from build123d import *

# Parameters (mm, degrees)
BOSS_EXTRUDE1_DEPTH = 3
FILLET4_R           = 0.7
FILLET5_R           = 4.8


with BuildPart() as part:
    # Sketch1 → Boss-Extrude1 (new body)
    with BuildSketch(Plane(origin=(0, 0, 0), x_dir=(1, 0, 0), z_dir=(0, 1, 0))):
        Polygon((-25, -25), (25, -25), (25, 20.2), (20.2, 20.2), (20.2, 3.75), (16.600191324, 3.712885357), (16.528023963, 10.712513338), (13.028209972, 10.676429657), (8.674837116, 6.131306471), (8.798552593, -5.868055782), (13.244712056, -10.322454286), (16.744526047, -10.286370605), (16.672358686, -3.286742624), (20.272167361, -3.249627981), (20.272167361, -20.078881527), (3.743734852, -20.078881527), (3.725177284, -16.478929358), (10.725084279, -16.442845198), (10.707042199, -12.942891701), (6.184420516, -8.566147121), (-5.815420046, -8.628005682), (-10.292678785, -13.051144181), (-10.274636705, -16.551097679), (-3.27472971, -16.515013518), (-3.256172142, -20.114965687), (-20, -20.114965687), (-20, -3.5), (-16.4, -3.5), (-16.4, -10.5), (-12.9, -10.5), (-8.5, -6), (-8.5, 6), (-12.9, 10.5), (-16.4, 10.5), (-16.4, 3.5), (-20, 3.5), (-20, 20.2), (-25, 20.2), align=None)
    extrude(amount=BOSS_EXTRUDE1_DEPTH)

    # Fillet4
    fillet4_edges = [part.edges().sort_by_distance(p)[0] for p in [
        (-3.27472971, 1.5, 16.515013518),
        (-10.274636705, 1.5, 16.551097679),
        (-10.292678785, 1.5, 13.051144181),
        (10.707042199, 1.5, 12.942891701),
        (10.725084279, 1.5, 16.442845198),
        (3.725177284, 1.5, 16.478929358),
        (3.743734852, 1.5, 20.078881527),
        (20.272167361, 1.5, 3.249627981),
        (16.672358686, 1.5, 3.286742624),
        (16.744526047, 1.5, 10.286370605),
        (13.244712056, 1.5, 10.322454286),
        (13.028209972, 1.5, -10.676429657),
        (16.528023963, 1.5, -10.712513338),
        (16.600191324, 1.5, -3.712885357),
        (20.2, 1.5, -3.75),
        (-20, 1.5, -3.5),
        (-16.4, 1.5, -3.5),
        (-16.4, 1.5, -10.5),
        (-12.9, 1.5, -10.5),
        (-12.9, 1.5, 10.5),
        (-16.4, 1.5, 10.5),
        (-16.4, 1.5, 3.5),
        (-20, 1.5, 3.5),
        (-3.256172142, 1.5, 20.114965687),
    ]]
    fillet(fillet4_edges, radius=FILLET4_R)

    # Fillet5
    fillet5_edges = [part.edges().sort_by_distance(p)[0] for p in [
        (-5.815420046, 1.5, 8.628005682),
        (6.184420516, 1.5, 8.566147121),
        (8.798552593, 1.5, 5.868055782),
        (8.674837116, 1.5, -6.131306471),
        (-8.5, 1.5, -6),
        (-8.5, 1.5, 6),
    ]]
    fillet(fillet5_edges, radius=FILLET5_R)


solid = part.part
Verification items for the finished model (mm, model axes). A direction names the side the tool comes from. Coordinates: 2 decimals unless noted, no trailing zeros. Order: outer loops, then holes, each group sorted by start corner. A loop starts at its lowest first (then second) coordinate and runs counter-clockwise, first axis right, second up. Notation, with made-up numbers: (26.25, -32) -> (72.25, -32) arc R32 ccw to (72.25, 3) -> close; hole circle Ø6 at (67, 16.25). An arc over 180 degrees is marked (long way). Put each result on its own line as item: value. Start each with the question number.
1. Mould release check, pull along Z, two halves, no side actions. Record for faces 1 (the flat face through (-18, 1, -3.5)), 2 (the flat face through (-20, 1, 12)), 3 (the flat face through (-25, 1, 2)): released by +Z, released by -Z, zero draft, split by the parting line, or undercut.
2. Go/stop test with flat-tipped pins: pin 1 Ø0.9 at (x, y) = (12.5, 1.5) entering from -Z; pin 2 Ø2 at (x, z) = (16, -4.5) entering from -Y; pin 3 Ø0.8 at (x, y) = (-14.5, 1) entering from -Z; pin 4 Ø1.1 at (x, y) = (-18.5, 2) entering from -Z. Record where each tip stops, or that it passes through.
3. Cross-section at A-A, the plane z = -17. Record the boundary of the cut face in (x, y), then the cut area to 3 significant figures.
4. Material ranges on L1, parallel to X at y = 0.8, z = 15; L2, parallel to X at y = 1.8, z = 13; L3, parallel to Z at x = -13.5, y = 0.5, recorded low to high. Write a range as [from, to].
5. Access from +Z, -Z, +X, -X, +Y, -Y to the whole of each face (thin tool, end or side, straight path). Record for faces 4 (the flat face through (12, 1, 20.079)), 5 (the flat face through (20.2, 1, -12)), 6 (the flat face through (25, 1, 3)).
6. Cross-section at B-B, the plane x = -15. Record the boundary of the cut face in (y, z).
Computed:
1. face 1: released by -Z
1. face 2: undercut
1. face 3: zero draft
2. pin 1: z = -10.57
2. pin 2: y = 0
2. pin 3: z = -10.5
2. pin 4: z = -3.5
3. outline: (-25, 0) -> (-20, 0) -> (-20, 3) -> (-25, 3) -> close; (20.2, 0) -> (25, 0) -> (25, 3) -> (20.2, 3) -> close
3. area: 29.4 mm2
4. L1: [-25, -20], [-10.28, 10.72], [20.27, 25]
4. L2: [-25, -20], [-10.2, 10.67], [20.27, 25]
4. L3: [-10.5, 10.5], [20.11, 25]
5. face 4: +Y, -Y
5. face 5: -Z, +Y, -Y
5. face 6: +Z, -Z, +X, +Y, -Y
6. outline: (0, -10.5) -> (3, -10.5) -> (3, 10.5) -> (0, 10.5) -> close; (0, 20.11) -> (3, 20.11) -> (3, 25) -> (0, 25) -> close
